```python
from build123d import *

# Parameters (mm, degrees)
TILT_MOUNT_DEPTH              = 11.938
SERVO_HOLE_SKETCH_W           = 27.94
SERVO_HOLE_SKETCH_H           = 13.208
SERVO_HOLE_DEPTH              = 12.938
MOUNTING_HOLES_GUIDE_SKETCH_R = 1.778
MOUNTING_HOLES_DEPTH          = 12.938


with BuildPart() as part:
    # Tilt Mount Sketch → Tilt Mount (new body)
    with BuildSketch(Plane(origin=(0, 0, 0), x_dir=(1, 0, 0), z_dir=(0, 1, 0))):
        Polygon((44.45, 0), (50.8, 0), (50.8, 25.4), (0, 25.4), (0, 0), (6.35, 0), (6.35, -11.938), (44.45, -11.938), align=None)
    extrude(amount=TILT_MOUNT_DEPTH)

    # Servo Hole Sketch → Servo Hole (cut, through all)
    with BuildSketch(Plane(origin=(0, 11.938, 0), x_dir=(1, 0, 0), z_dir=(0, 1, 0))):
        with Locations((25.4, 12.954)):
            Rectangle(SERVO_HOLE_SKETCH_W, SERVO_HOLE_SKETCH_H)
    extrude(amount=-SERVO_HOLE_DEPTH, mode=Mode.SUBTRACT)

    # Mounting Holes Guide Sketch → Mounting Holes (cut, through all)
    with BuildSketch(Plane(origin=(0, 11.938, 0), x_dir=(1, 0, 0), z_dir=(0, 1, 0))):
        with Locations((8.636, 12.954)):
            Circle(MOUNTING_HOLES_GUIDE_SKETCH_R)
        with Locations((42.164, 12.954)):
            Circle(MOUNTING_HOLES_GUIDE_SKETCH_R)
    extrude(amount=-MOUNTING_HOLES_DEPTH, mode=Mode.SUBTRACT)


solid = part.part
```
Could you check a few things on this model? Use its own coordinates, in mm. A direction names the side the tool comes from. Round coordinates to 2 decimals unless told otherwise and drop trailing zeros. Write each loop counter-clockwise with the first axis right and the second up, starting at its lowest first coordinate (ties: lowest second). Pieces come first, ordered by that corner, then holes. Notation, with made-up numbers: M 75.5,8 L 120.5,8 A23 cw 120.5,47 Z; hole C 68,30 d3. An arc over 180 degrees is marked long. Answer in a Markdown table with one row per item. Add a question column.
Q1. Imagine slicing it at C-C (y = 11). Please give me the cut outline in (x, z).
Q2. If I drill on line 1 (X direction, y = 5.25, z = -18); line 2 (Z direction, x = 25, y = 5.25); line 3 (X direction, y = 10.5, z = 6), over which ranges is the centre line in solid material (lowest first)? Write a range as from..to.
Q3. Will these pins go through, and if not, where does the flat tip stop? pin 1 Ø6 at (y, z) = (6, 8.5) entering from +X; pin 2 Ø3 at (x, z) = (14, -20) entering from -Y; pin 3 Ø5 at (x, y) = (47.5, 4.5) entering from +Z.
Q4. If we mould it in two halves opening along X, with no side actions, what happens to faces 6 (the flat face through (39.37, 6, -13)), 7 (the flat face through (26, 6, -25.4)), 8 (the flat face through (50.8, 6, -13)), 9 (the flat face through (6.35, 6, 6))? For each: +X half, -X half, draft (parallel to the pull), parting line (faces both ways), or undercut.
Q5. Imagine slicing it at D-D (z = 6.5). Please give me the cut outline in (x, y), then the cut area to 3 significant figures.
Q6. On a 3-axis mill with a long thin cutter (end or side, diameter ignored), from which of +Z, -Z, +X, -X, +Y, -Y can I reach the whole of each face in a straight line? I mean faces 1 (the flat face through (25, 6, -19.558)), 2 (the flat face through (3, 6, 0)), 3 (the flat face through (25, 0, -3)), 4 (the flat face through (48, 6, 0)), 5 (the flat face through (25, 11.938, -3)). Say none if no direction works.
Q7. Imagine slicing it at A-A (z = -9). Please give me the cut outline in (x, y).
Q8. Imagine slicing it at B-B (x = 30). Please give me the cut outline in (y, z), then the cut area to 3 significant figures.
Values:
| question | item | result |
|---|---|---|
| 1 | outline | M 0,-25.4 L 50.8,-25.4 L 50.8,0 L 44.45,0 L 44.45,11.94 L 6.35,11.94 L 6.35,0 L 0,0 Z; hole C 8.64,-12.95 d3.56; hole M 11.43,-19.56 L 39.37,-19.56 L 39.37,-6.35 L 11.43,-6.35 Z; hole C 42.16,-12.95 d3.56 |
| 2 | line 1 | 0..11.43, 39.37..50.8 |
| 2 | line 2 | -25.4..-19.56, -6.35..11.94 |
| 2 | line 3 | 6.35..44.45 |
| 3 | pin 1 | x = 44.45 |
| 3 | pin 2 | y = 0 |
| 3 | pin 3 | z = 0 |
| 4 | face 6 | undercut |
| 4 | face 7 | draft |
| 4 | face 8 | +X half |
| 4 | face 9 | -X half |
| 5 | outline | M 6.35,0 L 44.45,0 L 44.45,11.94 L 6.35,11.94 Z |
| 5 | area | 455 mm^2 |
| 6 | face 1 | +Y, -Y |
| 6 | face 2 | +Z, -X, +Y, -Y |
| 6 | face 3 | +Z, -Z, +X, -X, -Y |
| 6 | face 4 | +Z, +X, +Y, -Y |
| 6 | face 5 | +Z, -Z, +X, -X, +Y |
| 7 | outline | M 0,0 L 11.43,0 L 11.43,11.94 L 0,11.94 Z; M 39.37,0 L 50.8,0 L 50.8,11.94 L 39.37,11.94 Z |
| 8 | outline | M 0,-25.4 L 11.94,-25.4 L 11.94,-19.56 L 0,-19.56 Z; M 0,-6.35 L 11.94,-6.35 L 11.94,11.94 L 0,11.94 Z |
| 8 | area | 288 mm^2 |
